```python
from build123d import *

# Parameters (mm, degrees)
FILLET1_R = 10


with BuildPart() as part:
    # Sketch2 → Revolve1 (revolve)
    with BuildSketch(Plane.XY):
        with BuildLine():
            Line((0, 0), (1.5, 0))
            Line((1.5, 0), (1.5, -3))
            Line((1.5, -3), (1.25, -6))
            Line((1.25, -6), (1.25, -47.272821971))
            ThreePointArc((1.25, -47.272821971), (2.931001031, -50.639713183), (0, -53))
            Line((0, -53), (0, 0))
        make_face()
    revolve(axis=Axis((0, -214.104441575, 0), (0, 1, 0)))

    # Fillet1
    # the kernel refuses this fillet: 10 mm, written as the material it adds along each edge
    with BuildSketch(Plane(origin=(0, -6, 0), x_dir=(1, 0, 0), z_dir=(0, 0, 1))) as fillet1_piece_1:
        with BuildLine():
            CenterArc((1.25 + FILLET1_R, -FILLET1_R * 0.0415945787923), FILLET1_R, 175.236358309, 4.763641691)
            Line((1.25, -FILLET1_R * 0.0415945787923), (1.25, 0))
            Line((1.25, 0), (1.25 + FILLET1_R * 0.00345424175512, FILLET1_R * 0.0414509010614))
        make_face()
    revolve(axis=Axis((0, -6, 0), (0, 1, 0)))
    # the kernel refuses this fillet: 10 mm, written as the material it takes off along each edge
    with BuildSketch(Plane(origin=(0, -3, 0), x_dir=(1, 0, 0), z_dir=(0, 0, 1))) as fillet1_2_piece_1:
        with BuildLine():
            CenterArc((1.5 - FILLET1_R, FILLET1_R * 0.0415945787923), FILLET1_R, 355.236358309, 4.763641691)
            Line((1.5 - FILLET1_R * 0.00345424175512, -FILLET1_R * 0.0414509010614), (1.5, 0))
            Line((1.5, 0), (1.5, FILLET1_R * 0.0415945787923))
        make_face()
    revolve(axis=Axis((0, -3, 0), (0, 1, 0)), mode=Mode.SUBTRACT)


solid = part.part
```
Can you work these out from the model? Positions are in its coordinate system, mm. Coordinates: 2 decimals unless noted, no trailing zeros. Write each loop counter-clockwise with the first axis right and the second up, starting at its lowest first coordinate (ties: lowest second). Pieces come first, ordered by that corner, then holes. Notation, with made-up numbers: (-29.75, 12) - (-14.75, 12) arc R21 ccw to (-14.75, 48) - close; hole circle Ø2 at (66, -26). An arc over 180 degrees is marked (long way). Return JSON: item names as keys, results as strings.
Q1. Thinking about a two-plate mould opening in Y: for faces 1 (the cylindrical face through (-0.27, -27.13, 1.22)), 2 (the cylindrical face through (-1.5, -1.31, -0.07)), 3 (the flat face through (0, 0, 0)), which applies, +Y half, -Y half, draft (parallel to the pull), parting line (faces both ways), or undercut?
Computed values:
{"face 1": "undercut", "face 2": "draft", "face 3": "+Y half"}
Q2. Please list where these lines run through material, in increasing order: L1, parallel to X at y = -47, z = 0; L2, parallel to Y at x = -1.75, z = 1. Write a range as from..to.
Computed values:
{"L1": "x = -1.25..1.25", "L2": "y = -52.22..-47.78"}
Q3. If we section it at A-A (y = -32.5): Please give me the cut outline in (x, z), then the cut area to 3 significant figures.
Computed values:
{"outline": "circle Ø2.5 at (0, 0)", "area": "4.91 mm2"}
Q4. If we section it at B-B (y = -50): Please give me the cut outline in (x, z).
Computed values:
{"outline": "circle Ø6 at (0, 0)"}
Q5. I'm going to push flat-ended pins straight in: pin 1 Ø1.5 at (x, y) = (-1, -14) entering from -Z; pin 2 Ø1 at (y, z) = (-6, 1.5) entering from -X; pin 3 Ø1 at (y, z) = (-43, 1.5) entering from -X. Where does each tip first touch, or does it pass through?
Computed values:
{"pin 1": "stops at z = -1.22", "pin 2": "stops at x = -0.77", "pin 3": "stops at x = -0.75"}
